```python
from build123d import *

# Parameters (mm, degrees)
BOSS_EXTRUDE1_DEPTH                             = 4
SKETCH2_R                                       = 35.885499984
SKETCH2_R_2                                     = 27.94
BOSS_EXTRUDE2_DEPTH                             = 15.24
SKETCH5_W                                       = 2.8067
SKETCH5_H                                       = 4.953
SKETCH10_W                                      = 10.702500058
SKETCH10_H                                      = 79.03151748
CUT_EXTRUDE2_DEPTH                              = 72.905773325
CSK_FOR_M3_FLAT_HEAD_MACHINE_SCREW1_D           = 3.4
CSK_FOR_M3_FLAT_HEAD_MACHINE_SCREW1_CSINK_D     = 7
CSK_FOR_M3_FLAT_HEAD_MACHINE_SCREW1_CSINK_ANGLE = 90


with BuildPart() as part:
    # Sketch1 → Boss-Extrude1 (new body)
    with BuildSketch(Plane(origin=(0, 0, 0), x_dir=(1, 0, 0), z_dir=(0, 1, 0))):
        with BuildLine():
            Line((-48.446276818, 28.421125), (-48.446276818, 0))
            Line((-48.446276818, 0), (41.648, 0))
            ThreePointArc((41.648, 0), (7.018876975, 47.235418548), (-48.446276818, 28.421125))
        make_face()
        with BuildLine():
            Line((41.648, 0), (-48.446276818, 0))
            Line((-48.446276818, 0), (-48.446276818, -28.421125))
            ThreePointArc((-48.446276818, -28.421125), (7.018876975, -47.235418548), (41.648, 0))
        make_face()
    extrude(amount=BOSS_EXTRUDE1_DEPTH)

    # Sketch2 → Boss-Extrude2 (add)
    with BuildSketch(Plane(origin=(0, 4, 0), x_dir=(1, 0, 0), z_dir=(0, 1, 0))):
        with Locations(Location((0, 0, 0), (0, 0, 90))):
            Circle(SKETCH2_R)
        with Locations(Location((0, 0, 0), (0, 0, 90))):
            Circle(SKETCH2_R_2, mode=Mode.SUBTRACT)
    extrude(amount=BOSS_EXTRUDE2_DEPTH)

    # Sketch5 → Cut-Revolve1 (revolve, cut)
    with BuildSketch(Plane(origin=(0, 0, 0), x_dir=(0, 0, -1), z_dir=(1, 0, 0)), mode=Mode.PRIVATE) as cut_revolve1_sk:
        with Locations((-34.482149984, 8.064)):
            Rectangle(SKETCH5_W, SKETCH5_H)
        with Locations((-34.482149984, 15.176)):
            Rectangle(SKETCH5_W, SKETCH5_H)
    revolve(cut_revolve1_sk.sketch.rotate(Axis((0, 19.24, 0), (0, -1, 0)), 180), axis=Axis((0, 19.24, 0), (0, -1, 0)), mode=Mode.SUBTRACT)

    # Sketch10 → Cut-Extrude2 (cut, through all)
    with BuildSketch(Plane.XZ):
        with Locations((-43.095026789, 0)):
            Rectangle(SKETCH10_W, SKETCH10_H)
    extrude(amount=-CUT_EXTRUDE2_DEPTH, mode=Mode.SUBTRACT)

    # CSK for M3 Flat Head Machine Screw1 (through all)
    with Locations(Plane(origin=(0, 0, 0), x_dir=(-1, 0, 0), z_dir=(0, -1, 0))):
        with Locations((26.932, -40.64), (-11.168, -40.64), (-11.168, 40.64), (26.932, 40.64)):
            CounterSinkHole(CSK_FOR_M3_FLAT_HEAD_MACHINE_SCREW1_D / 2, CSK_FOR_M3_FLAT_HEAD_MACHINE_SCREW1_CSINK_D / 2, counter_sink_angle=CSK_FOR_M3_FLAT_HEAD_MACHINE_SCREW1_CSINK_ANGLE)


solid = part.part
```
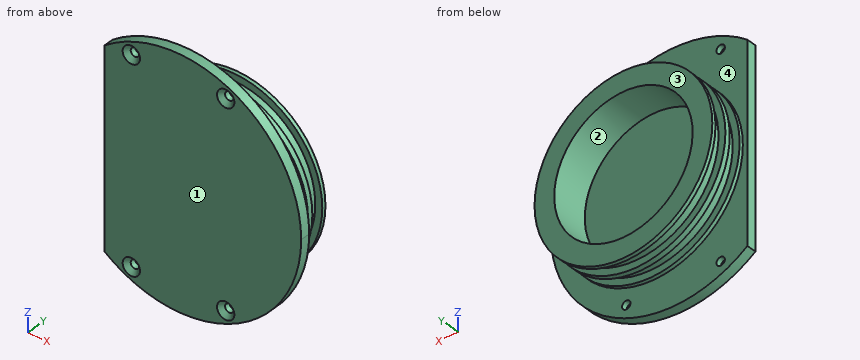
Model file for the job. Use its own axes, mm. Face numbers are marked on the shaded views. A direction names the side the tool comes from. Coordinates: 2 decimals unless noted, no trailing zeros. Loops run counter-clockwise (first coordinate to the right, second up) from the corner with the lowest first, then second, coordinate; pieces in that order, holes last. Notation, with made-up numbers: (-29, 35.25) -> (-4, 35.25) arc R28 cw to (-4, 72.25) -> close; hole circle Ø9 at (62, 8). An arc over 180 degrees is marked (long way). Answer as a JSON object with one key per item and string values.
Q1. Cut at D-D (z = 2.5). List the corners of the cut face in (x, y), and give its area (4 significant figures).
Report:
{"outline": "(-37.74, 0) -> (41.58, 0) -> (41.58, 4) -> (35.8, 4) -> (35.8, 5.59) -> (32.98, 5.59) -> (32.98, 10.54) -> (35.8, 10.54) -> (35.8, 12.7) -> (32.98, 12.7) -> (32.98, 17.65) -> (35.8, 17.65) -> (35.8, 19.24) -> (27.83, 19.24) -> (27.83, 4) -> (-27.83, 4) -> (-27.83, 19.24) -> (-35.8, 19.24) -> (-35.8, 17.65) -> (-32.98, 17.65) -> (-32.98, 12.7) -> (-35.8, 12.7) -> (-35.8, 10.54) -> (-32.98, 10.54) -> (-32.98, 5.59) -> (-35.8, 5.59) -> (-35.8, 4) -> (-37.74, 4) -> close", "area": "504.5 mm2"}
Q2. Probe probe 1 along Y at (x, z) = (31, 14); probe 2 along Z at (x, y) = (-1, 9.75); probe 3 along Y at (x, z) = (-31.5, -43). List the from-to ranges inside material, lowest first.
Report:
{"probe 1": "y = 0 to 5.59, 10.54 to 12.7, 17.65 to 19.24", "probe 2": "z = -33.06 to -27.92, 27.92 to 33.06", "probe 3": "y = 0 to 4"}
Q3. Cut at B-B (z = 40.64). List the corners of the cut face in (x, y), and give its area (3 significant figures).
Report:
{"outline": "(-36.19, 0) -> (-30.43, 0) -> (-28.63, 1.8) -> (-28.63, 4) -> (-36.19, 4) -> close; (-25.23, 1.8) -> (-23.43, 0) -> (7.67, 0) -> (9.47, 1.8) -> (9.47, 4) -> (-25.23, 4) -> close; (12.87, 1.8) -> (14.67, 0) -> (20.43, 0) -> (20.43, 4) -> (12.87, 4) -> close", "area": "193 mm2"}
Q4. 3-axis set-ups, long thin cutter, end or side, ignore diameter. For the marked faces 3 and 4: which of +Z, -Z, +X, -X, +Y, -Y reach the whole face in a straight line?
Report:
{"face 3": "+Z, -Z, +X, -X, +Y", "face 4": "+Y"}
Q5. Cut at A-A (y = 16.5). List the corners of the cut face in (x, z), and give its area (3 significant figures).
Report:
{"outline": "circle Ø66.16 at (0, 0); hole circle Ø55.88 at (0, 0)", "area": "985 mm2"}
Q6. Pull direction Z, two halves, no side cores. Call the marked faces 1 and 2: released by +Z, released by -Z, zero draft, split by the parting line, or undercut.
Report:
{"face 1": "zero draft", "face 2": "undercut"}
Q7. Flat gauge pins, fed straight in: P1, Ø10, axis at x = 2.5, y = 12.5, coming from the -Z side; P2, Ø4, axis at x = -25, y = 12.5, coming from the +Z side; P3, Ø3, axis at x = -12, y = 3, coming from the +Z side. Where does each tip first touch, or does it go through?
Report:
{"P1": "stops at z = -35.89", "P2": "stops at z = 27.55", "P3": "stops at z = 49.46"}
Q8. Cut at C-C (x = 0). List the corners of the cut face in (y, z), and give its area (3 significant figures).
Report:
{"outline": "(0, -48.9) -> (4, -48.9) -> (4, -35.89) -> (5.59, -35.89) -> (5.59, -33.08) -> (10.54, -33.08) -> (10.54, -35.89) -> (12.7, -35.89) -> (12.7, -33.08) -> (17.65, -33.08) -> (17.65, -35.89) -> (19.24, -35.89) -> (19.24, -27.94) -> (4, -27.94) -> (4, 27.94) -> (19.24, 27.94) -> (19.24, 35.89) -> (17.65, 35.89) -> (17.65, 33.08) -> (12.7, 33.08) -> (12.7, 35.89) -> (10.54, 35.89) -> (10.54, 33.08) -> (5.59, 33.08) -> (5.59, 35.89) -> (4, 35.89) -> (4, 48.9) -> (0, 48.9) -> close", "area": "578 mm2"}
